For this review, use the dimensioned drawing (mm, ordinates from the lowest corner) and the shaded views. A direction names the side the tool comes from. Give positions to 0.01 mm unless a question says otherwise; leave off trailing zeros. Order: outer loops, then holes, each group sorted by start corner. A loop starts at its lowest first (then second) coordinate and runs counter-clockwise, first axis right, second up. Notation, with made-up numbers: (-3, -34.5) - (12, -34.5) arc R28 cw to (12, -13.5) - close; hole circle Ø3 at (12, -31). An arc over 180 degrees is marked (long way). Use a Markdown table: item, result. Add a question column.
1) Clearance check with flat-ended pins moving along their axes: P1, Ø2.5, axis at x = 6, y = 12, coming from the +Z side; P2, Ø3.5, axis at x = 3, y = 3, coming from the -Z side; P3, Ø8, axis at y = 12.5, z = 4, coming from the +X side; P4, Ø1.7, axis at x = 9, y = 3, coming from the +Z side. State where each tip first meets the part, or that it passes through.
2) We need section B-B on y = 12. Write out the cut boundary in (x, z).
3) We need section C-C on z = 1. Write out the cut boundary in (x, y).
4) We need section D-D on y = 3. Write out the cut boundary in (x, z).
5) Machinability: for the marked faces 1, 2 and 3, which of the approach directions +Z, -Z, +X, -X, +Y, -Y give a long, thin tool a straight path to every point of the face, cutting with its end or side? Answer none if there is none.
6) Mouldability with a two-part tool opening along Y and no side actions: class the marked faces 4, 5 and 6 as released by +Y, released by -Y, zero draft, split by the parting line, or undercut.
7) Wall thickness on L1, parallel to Y at x = 9, z = 14.25; L2, parallel to Z at x = 3.25, y = 10.5; L3, parallel to Z at x = 7, y = 6.75: over which ranges is each line inside the solid? List them lowest first.
8) We need section A-A on x = 6. Write out the cut boundary in (y, z), then the cut area to 3 significant figures.
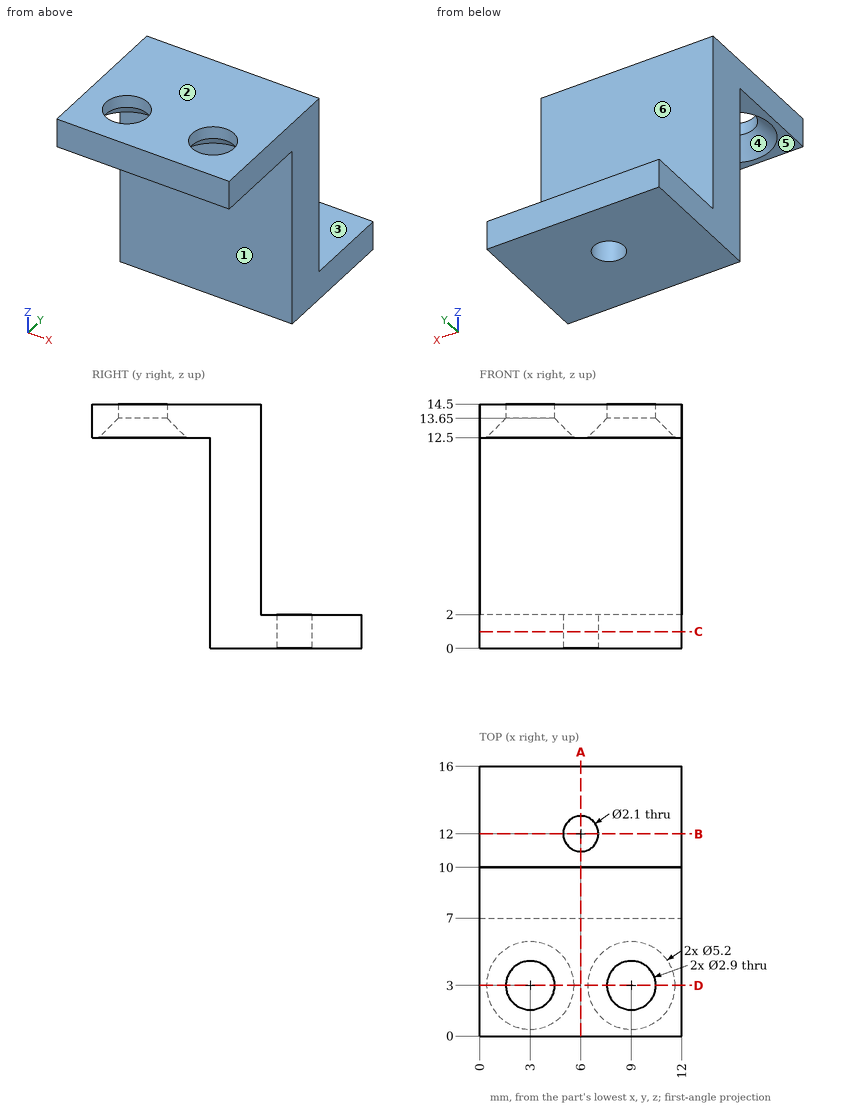
Checked values:
| question | item | result |
|---|---|---|
| 1 | P1 | z = 2 |
| 1 | P2 | z = 13.35 |
| 1 | P3 | x = 12 |
| 1 | P4 | through |
| 2 | outline | (0, 0) - (4.95, 0) - (4.95, 2) - (0, 2) - close; (7.05, 0) - (12, 0) - (12, 2) - (7.05, 2) - close |
| 3 | outline | (0, 7) - (12, 7) - (12, 16) - (0, 16) - close; hole circle Ø2.1 at (6, 12) |
| 4 | outline | (0, 12.5) - (0.4, 12.5) - (1.55, 13.65) - (1.55, 14.5) - (0, 14.5) - close; (4.45, 13.65) - (5.6, 12.5) - (6.4, 12.5) - (7.55, 13.65) - (7.55, 14.5) - (4.45, 14.5) - close; (10.45, 13.65) - (11.6, 12.5) - (12, 12.5) - (12, 14.5) - (10.45, 14.5) - close |
| 5 | face 1 | -Z, +X, -X, -Y |
| 5 | face 2 | +Z, +X, -X, +Y, -Y |
| 5 | face 3 | +Z, +X, -X, +Y |
| 6 | face 4 | undercut |
| 6 | face 5 | zero draft |
| 6 | face 6 | released by +Y |
| 7 | L1 | 0 to 1.55, 4.45 to 10 |
| 7 | L2 | 0 to 2 |
| 7 | L3 | 12.5 to 14.5 |
| 8 | outline | (0, 12.5) - (7, 12.5) - (7, 0) - (10.95, 0) - (10.95, 2) - (10, 2) - (10, 14.5) - (0, 14.5) - close; (13.05, 0) - (16, 0) - (16, 2) - (13.05, 2) - close |
| 8 | area | 65.3 mm² |
